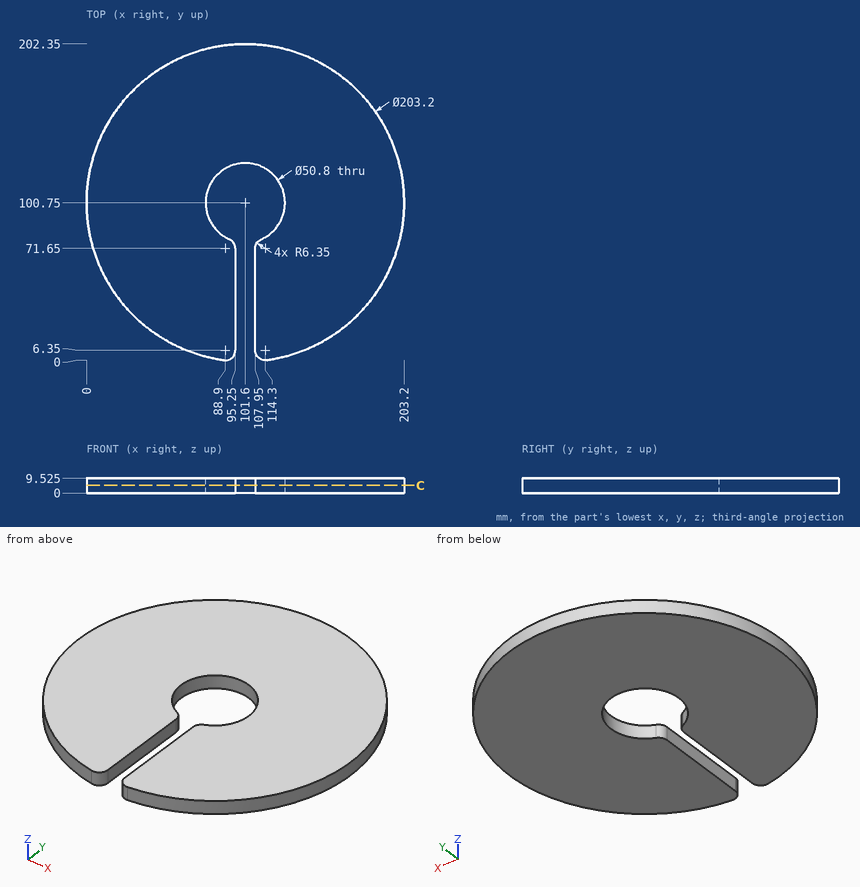
The figure shows three views and two pictorial views of one solid part (mm, origin at its lowest corner). Answer the questions. Round coordinates to 2 decimals unless told otherwise and drop trailing zeros. Write each loop counter-clockwise with the first axis right and the second up, starting at its lowest first coordinate (ties: lowest second). Pieces come first, ordered by that corner, then holes. Notation, with made-up numbers: M 71,3.5 L 82,3.5 A11 ccw 82,24.5 Z; hole C 61,-28 d6. An arc over 180 degrees is marked long. Write each question's results on one line, items separated by ' | '. Start each with the question number.
(1) Each of these flat-tipped pins is pushed along its axis until it touches: P1, Ø1, axis at x = 46, z = 2.5, coming from the +Y side; P2, Ø3, axis at y = 50, z = 6, coming from the -X side (1 decimal); P3, Ø5, axis at y = 31, z = 4.5, coming from the +X side. Where does it stop, or does it pass through?
(2) The part is cut by section C-C, the plane z = 5. Write down the section's boundary in (x, y).
(3) Find the intervals of material crossed by line 1 (X direction, y = 26.5, z = 4.5); line 2 (Y direction, x = 101.6, z = 5.25); line 3 (Y direction, x = 115, z = 4.75), in increasing order.
Worked answers:
1) P1: stops at y = 186.11 | P2: stops at x = 12.7 | P3: stops at x = 177.76
2) outline: M 88.05,0.06 A6.35 ccw 95.25,6.35 L 95.25,71.65 A6.35 ccw 91.44,77.47 A25.4 cw long 111.76,77.47 A6.35 ccw 107.95,71.65 L 107.95,6.35 A6.35 ccw 115.15,0.06 A101.6 ccw long Z
3) line 1: x = 32.25 to 95.25, 107.95 to 170.95 | line 2: y = 126.15 to 202.35 | line 3: y = 0.04 to 79.17, 122.33 to 201.46
